```python
from build123d import *

# Parameters (mm, degrees)
F0_W      = 210
F0_H      = 180
F1_DEPTH  = 30
F2_W      = 202
F2_H      = 175
F3_DEPTH  = 28
F4_R      = 3
F5_DEPTH  = 4
F6_W      = 10
F6_H      = 82.5
F6_W_2    = 20
F6_H_2    = 10
F6_W_3    = 142
F7_DEPTH  = 2
F8_R      = 2
F9_DEPTH  = 5
F10_R     = 2
F10_R_2   = 7.5
F11_DEPTH = 5
F12_R     = 7.5
F13_DEPTH = 5
F14_W     = 8
F14_H     = 20
F15_DEPTH = 25
F17_DEPTH = 5
F19_DEPTH = 5
F21_DEPTH = 5
F23_DEPTH = 5
F25_DEPTH = 5
F27_DEPTH = 5
F30_DEPTH = 5
F32_DEPTH = 5
F33_R     = 3
F34_DEPTH = 4


# Not quite as in the source:
# - a feature names something its author has since deleted; it is built from what else it names


with BuildPart() as f1:
    # F0 (on Top) → F1 (new body)
    with BuildSketch(Plane.XY):
        Rectangle(F0_W, F0_H)
    extrude(amount=F1_DEPTH)

    # F2 (on face) → F3 (cut)
    with BuildSketch(Plane.XY.offset(30)):
        Rectangle(F2_W, F2_H)
    extrude(amount=-F3_DEPTH, mode=Mode.SUBTRACT)

    # F4 (on face) → F5 (cut)
    with BuildSketch(Plane.XZ.offset(90)):
        with BuildLine():
            Line((-57, 10), (-15, 10))
            Line((-15, 10), (15, 10))
            Line((15, 10), (57, 10))
            ThreePointArc((57, 10), (62.6568542495, 12.3431457505), (65, 18))
            Line((65, 18), (65, 30))
            Line((65, 30), (-65, 30))
            Line((-65, 30), (-65, 18))
            ThreePointArc((-65, 18), (-62.6568542495, 12.3431457505), (-57, 10))
        make_face()
        with Locations((-75, 15)):
            Circle(F4_R)
        with Locations((75, 15)):
            Circle(F4_R)
    extrude(amount=-F5_DEPTH, mode=Mode.SUBTRACT)

    # F8 (on face) → F9 (cut)
    with BuildSketch(Plane.YZ.offset(105)):
        with Locations((0, 15)):
            Circle(F8_R)
    extrude(amount=-F9_DEPTH, mode=Mode.SUBTRACT)

    # F10 (on face) → F11 (cut)
    with BuildSketch(Plane(origin=(-105, 0, 0), x_dir=(0, -1, 0), z_dir=(-1, 0, 0))):
        with Locations((0, 15)):
            Circle(F10_R)
        with Locations((-65, 15)):
            Circle(F10_R_2)
        with Locations((65, 15)):
            Circle(F10_R_2)
    extrude(amount=-F11_DEPTH, mode=Mode.SUBTRACT)

    # F12 (on face) → F13 (cut)
    with BuildSketch(Plane.YZ.offset(105)):
        with Locations((-66.0775899887, 15)):
            Circle(F12_R)
        with Locations((62.939658761, 15)):
            Circle(F12_R)
    extrude(amount=-F13_DEPTH, mode=Mode.SUBTRACT)

    # F14 (on face) → F15 (join)
    with BuildSketch(Plane.XY.offset(2)):
        with Locations((-97, 65)):
            Rectangle(F14_W, F14_H)
        with Locations((-97, -65)):
            Rectangle(F14_W, F14_H)
        with Locations((97, 65)):
            Rectangle(F14_W, F14_H)
        with Locations((97, -65)):
            Rectangle(F14_W, F14_H)
    extrude(amount=F15_DEPTH)

    # F16 (on face) → F17 (join)
    with BuildSketch(Plane(origin=(0, -55, 0), x_dir=(-1, 0, 0), z_dir=(0, 1, 0))):
        Polygon((-93, 2), (-81.6266089678, 1.707098214), (-93, 14.5), align=None)
    extrude(amount=-F17_DEPTH)

    # F18 (on face) → F19 (join)
    with BuildSketch(Plane.XZ.offset(-55)):
        Polygon((-93, 14.5), (-93, 2), (-81.0206457973, 2), align=None)
    extrude(amount=-F19_DEPTH)

    # F20 (on face) → F21 (join)
    with BuildSketch(Plane.XZ.offset(-55)):
        Polygon((81.1605315804, 2), (93, 2), (93, 14.5), align=None)
    extrude(amount=-F21_DEPTH)

    # F22 (on face) → F23 (join)
    with BuildSketch(Plane(origin=(0, -55, 0), x_dir=(-1, 0, 0), z_dir=(0, 1, 0))):
        Polygon((81.4045146108, 2), (93, 2), (93, 14.5), align=None)
    extrude(amount=-F23_DEPTH)

    # F24 (on face) → F25 (join)
    with BuildSketch(Plane(origin=(0, 75, 0), x_dir=(-1, 0, 0), z_dir=(0, 1, 0))):
        Polygon((81.214748323, 2), (93, 2), (93, 14.5), align=None)
    extrude(amount=-F25_DEPTH)

    # F26 (on face) → F27 (join)
    with BuildSketch(Plane.XZ.offset(75)):
        Polygon((81.2978520989, 2), (93, 2), (93, 14.5), align=None)
    extrude(amount=-F27_DEPTH)


with BuildPart() as f7:
    # F6 (on face) → F7 (new body)
    with BuildSketch(Plane.XY.offset(2)):
        with Locations((-76, 46.25)):
            Rectangle(F6_W, F6_H)
        with Locations((76, 46.25)):
            Rectangle(F6_W, F6_H)
        with Locations((-91, 0)):
            Rectangle(F6_W_2, F6_H_2)
        with Locations((-76, 0)):
            Rectangle(F6_W, F6_H_2)
        with Locations((-76, -46.25)):
            Rectangle(F6_W, F6_H)
        Rectangle(F6_W_3, F6_H_2)
        with Locations((76, 0)):
            Rectangle(F6_W, F6_H_2)
        with Locations((76, -46.25)):
            Rectangle(F6_W, F6_H)
        with Locations((91, 0)):
            Rectangle(F6_W_2, F6_H_2)
    extrude(amount=F7_DEPTH)


with BuildPart() as f1_1:
    add(f1.part)

    # F28: union F7
    add(f7.part)

    # F29 (on face) → F30 (join)
    with BuildSketch(Plane.XZ.offset(75)):
        Polygon((-93, 14.5), (-93, 2), (-81.4201831818, 2), align=None)
    extrude(amount=-F30_DEPTH)

    # F31 (on face) → F32 (join)
    with BuildSketch(Plane(origin=(0, 75, 0), x_dir=(-1, 0, 0), z_dir=(0, 1, 0))):
        Polygon((-93, 14.5), (-93, 2), (-81.2787339091, 2), align=None)
    extrude(amount=-F32_DEPTH)

    # F33 (on face) → F34 (cut)
    with BuildSketch(Plane(origin=(0, 90, 0), x_dir=(-1, 0, 0), z_dir=(0, 1, 0))):
        with BuildLine():
            Line((-57, 10.0647527289), (-15, 10.0647527289))
            Line((-15, 10.0647527289), (15, 10.0647527289))
            Line((15, 10.0647527289), (57, 10.0647527289))
            ThreePointArc((57, 10.0647527289), (62.6568542495, 12.4078984794), (65, 18.0647527289))
            Line((65, 18.0647527289), (65, 30))
            Line((65, 30), (-65, 30))
            Line((-65, 30), (-65, 18.0647527289))
            ThreePointArc((-65, 18.0647527289), (-62.6568542495, 12.4078984794), (-57, 10.0647527289))
        make_face()
        with Locations((-74.9857133275, 14.9857269089)):
            Circle(F33_R)
        with Locations((75, 15)):
            Circle(F33_R)
    extrude(amount=-F34_DEPTH, mode=Mode.SUBTRACT)


solid = f1_1.part
```
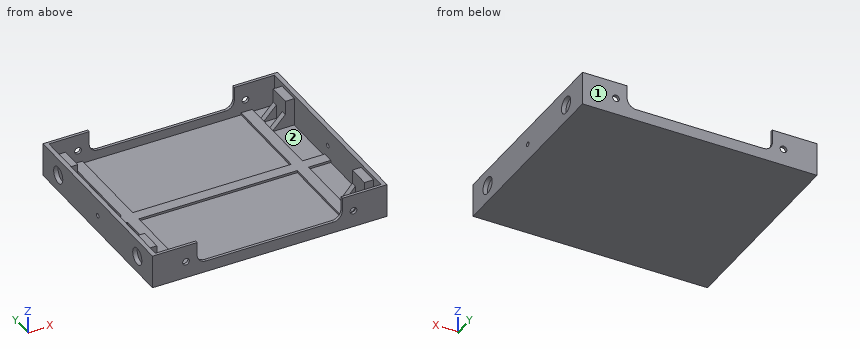
Input: part model. Units: mm. Frame: model coordinates. Face numbers are marked on the shaded views. A direction names the side the tool comes from. Coordinates: 2 decimals unless noted, no trailing zeros. Loops run counter-clockwise (first coordinate to the right, second up) from the corner with the lowest first, then second, coordinate; pieces in that order, holes last. Notation, with made-up numbers: (50, -33) - (98, -33) arc R24 cw to (98, -6) - close; hole circle Ø9 at (-23, -35.75). An arc over 180 degrees is marked (long way). Answer in a Markdown table with one row per item.
(1) Set-up query: the marked faces 1 and 2. Return all of +Z, -Z, +X, -X, +Y, -Y with unobstructed straight access to the full face (end or side cutting, diameter ignored); none if empty.
Model answer:
| item | result |
|---|---|
| face 1 | +Z, -Z, +X, -X, +Y |
| face 2 | +Z |
(2) Cut plane B-B on y = -27. Output: boundary loops of the cut face in (x, z).
Model answer:
| item | result |
|---|---|
| outline | (-105, 0) - (105, 0) - (105, 30) - (101, 30) - (101, 2) - (81, 2) - (81, 4) - (71, 4) - (71, 2) - (-71, 2) - (-71, 4) - (-81, 4) - (-81, 2) - (-101, 2) - (-101, 30) - (-105, 30) - close |
(3) Cut plane D-D on y = 65. Output: boundary loops of the cut face in (x, z).
Model answer:
| item | result |
|---|---|
| outline | (-105, 0) - (105, 0) - (105, 7.79) - (101, 7.79) - (101, 22.21) - (105, 22.21) - (105, 30) - (101, 30) - (101, 27) - (93, 27) - (93, 2) - (81, 2) - (81, 4) - (71, 4) - (71, 2) - (-71, 2) - (-71, 4) - (-81, 4) - (-81, 2) - (-93, 2) - (-93, 27) - (-101, 27) - (-101, 30) - (-105, 30) - (-105, 22.5) - (-101, 22.5) - (-101, 7.5) - (-105, 7.5) - close |
(4) Material intervals for L1, parallel to Y at x = -91, z = 4.25; L2, parallel to Y at x = -34.5, z = 2.5; L3, parallel to Z at x = -104, y = -65, sorted ascending. Write a range as from..to.
Model answer:
| item | result |
|---|---|
| L1 | y = -90..-87.5, -75..-70, -60..-55, 55..60, 70..75, 87.5..90 |
| L2 | y = -90..-87.5, -5..5, 87.5..90 |
| L3 | z = 0..7.5, 22.5..30 |
(5) Pin query (flat end, axial travel): P1, Ø7.5, axis at y = -65, z = 14, coming from the +X side; P2, Ø2, axis at x = 24, y = 14.5, coming from the +Z side; P3, Ø9, axis at x = 96, y = -67, coming from the +Z side. Return the tip coordinate at first contact, or that it passes through.
Model answer:
| item | result |
|---|---|
| P1 | stops at x = 101 |
| P2 | stops at z = 2 |
| P3 | stops at z = 27 |
(6) Cut plane C-C on x = 28. Output: boundary loops of the cut face in (y, z), plus the area to 3 significant figures.
Model answer:
| item | result |
|---|---|
| outline | (-90, 0) - (90, 0) - (90, 10.06) - (87.5, 10.06) - (87.5, 2) - (5, 2) - (5, 4) - (-5, 4) - (-5, 2) - (-87.5, 2) - (-87.5, 10) - (-90, 10) - close |
| area | 420 mm² |
(7) Cut plane A-A on x = 75. Output: boundary loops of the cut face in (y, z).
Model answer:
| item | result |
|---|---|
| outline | (-90, 0) - (90, 0) - (90, 11.99) - (87.5, 11.99) - (87.5, 4) - (-87.5, 4) - (-87.5, 12) - (-90, 12) - close; (-90, 18) - (-87.5, 18) - (-87.5, 30) - (-90, 30) - close; (87.5, 17.99) - (90, 17.99) - (90, 30) - (87.5, 30) - close |
